from build123d import *

# Parameters (mm, degrees)
F0_W     = 13
F0_H     = 41.843747
F1_DEPTH = 2
F2_R     = 1.5


with BuildPart() as f1:
    # F0 (on Top) → F1 (new body)
    with BuildSketch(Plane.XY):
        with Locations((-1.757174, 11.714493)):
            Rectangle(F0_W, F0_H)
    extrude(amount=F1_DEPTH)

    # F2
    f2_edges = [f1.edges().sort_by_distance(p)[0] for p in [
        (-1.757174, -9.20738, 2),
        (4.742826, 11.714494, 2),
        (-1.757174, 32.636367, 2),
    ]]
    fillet(f2_edges, radius=F2_R)


solid = f1.part
Model file for the job. Use its own axes, mm. Coordinates: 2 decimals unless noted, no trailing zeros. Order: outer loops, then holes, each group sorted by start corner. A loop starts at its lowest first (then second) coordinate and runs counter-clockwise, first axis right, second up. Notation, with made-up numbers: (27, -40) -> (83, -40) arc R8 cw to (83, -31) -> close; hole circle Ø3 at (11, 63). An arc over 180 degrees is marked (long way). Return JSON: item names as keys, results as strings. Group by question number.
Item 1: Saw through at A-A on y = 22.5. Write the cut outline in (x, z), then the cut area to 3 significant figures.
Item 2: Flat gauge pin, fed straight in: P1, Ø1.5, axis at x = -3.5, y = 28, coming from the -Z side. Where does the tip first touch, or does it go through?
Item 3: Wall check: line 1 along Y through (x, z) = (-5, 0.6); line 2 along X through (y, z) = (6, 0.65); line 3 along X through (y, z) = (24, 1.05). Give the ranges that are in metal, low to high. Write a range as [from, to].
Item 4: Saw through at B-B on z = 1.3. Write the cut outline in (x, y), then the cut area to 3 significant figures.
Values found:
{
 "1": {"outline": "(-8.26, 0) -> (4.74, 0) -> (4.74, 0.5) arc R1.5 ccw to (3.24, 2) -> (-8.26, 2) -> close", "area": "25.5 mm2"},
 "2": {"P1": "stops at z = 0"},
 "3": {"line 1": "y = [-9.2, 32.63]", "line 2": "x = [-8.26, 4.74]", "line 3": "x = [-8.26, 4.64]"},
 "4": {"outline": "(-8.26, -8.98) -> (4.51, -8.98) -> (4.51, 32.41) -> (-8.26, 32.41) -> close", "area": "528 mm2"}
}
